from build123d import *

# Parameters (mm, degrees)
EXTRUDE_1_DEPTH      = 6
SKETCH_2_R           = 11.05
SKETCH_2_R_2         = 1.6
SKETCH_2_R_3         = 2.55
CUT_EXTRUDE_1_DEPTH  = 7
EXTRUDE_2_DEPTH      = 6
SKETCH_3_R           = 2.1
SKETCH_3_W           = 7
SKETCH_3_H           = 6
CUT_EXTRUDE_11_DEPTH = 7
EXTRUDE_21_DEPTH     = 6
SKETCH_31_R          = 2.1
SKETCH_31_W          = 7
SKETCH_31_H          = 6
CUT_EXTRUDE_12_DEPTH = 7
EXTRUDE_24_DEPTH     = 6
SKETCH_34_R          = 2.1
SKETCH_34_W          = 7
SKETCH_34_H          = 6
CUT_EXTRUDE_15_DEPTH = 7


with BuildPart() as part:
    # Эскиз1 → Бобышка-Вытянуть1 (new body)
    with BuildSketch(Plane.XY):
        with BuildLine():
            Line((0, -293.846153846), (66, -293.846153846))
            Line((66, -293.846153846), (66, -368.846153846))
            ThreePointArc((66, -368.846153846), (63.071067812, -375.917221658), (56, -378.846153846))
            Line((56, -378.846153846), (0, -378.846153846))
            Line((0, -378.846153846), (0, -293.846153846))
        make_face()
    extrude(amount=-EXTRUDE_1_DEPTH)

    # Эскиз2 → Вырез-Вытянуть1 (cut, through all)
    with BuildSketch(Plane.XY):
        with Locations((29, -353.846153846)):
            Circle(SKETCH_2_R)
        with Locations((44.5, -369.346153846)):
            Circle(SKETCH_2_R_2)
        with Locations((13.5, -369.346153846)):
            Circle(SKETCH_2_R_2)
        with Locations((13.5, -338.346153846)):
            Circle(SKETCH_2_R_2)
        with Locations((44.5, -338.346153846)):
            Circle(SKETCH_2_R_2)
        with Locations((29, -323.846153846)):
            Circle(SKETCH_2_R_3)
    extrude(amount=-CUT_EXTRUDE_1_DEPTH, mode=Mode.SUBTRACT)

    # Эскиз21 → Бобышка-Вытянуть2 (add)
    with BuildSketch(Plane(origin=(16, -335.846153846, 0), x_dir=(0, 1, 0), z_dir=(0, 0, -1))):
        with BuildLine():
            Line((13, 53), (-13, 53))
            ThreePointArc((-13, 53), (-14.118033989, 52.736067977), (-15, 52))
            Line((-15, 52), (-16.2, 50.4))
            ThreePointArc((-16.2, 50.4), (-16.552786405, 50.105572809), (-17, 50))
            Line((-17, 50), (17, 50))
            ThreePointArc((17, 50), (16.552786405, 50.105572809), (16.2, 50.4))
            Line((16.2, 50.4), (15, 52))
            ThreePointArc((15, 52), (14.118033989, 52.736067977), (13, 53))
        make_face()
    extrude(amount=EXTRUDE_2_DEPTH)

    # Эскиз3 → Вырез-Вытянуть11 (cut, through all)
    with BuildSketch(Plane(origin=(16, -335.846153846, -6), x_dir=(0, 1, 0), z_dir=(0, 0, -1))):
        with Locations((0, 47)):
            Circle(SKETCH_3_R)
        with Locations((9.531849908, 47)):
            Rectangle(SKETCH_3_W, SKETCH_3_H)
        with Locations((-9.531849908, 47)):
            Rectangle(SKETCH_3_W, SKETCH_3_H)
    extrude(amount=-CUT_EXTRUDE_11_DEPTH, mode=Mode.SUBTRACT)

    # Эскиз22 → Бобышка-Вытянуть21 (add)
    with BuildSketch(Plane(origin=(50, -310.846153846, 0), x_dir=(0, -1, 0), z_dir=(0, 0, -1))):
        with BuildLine():
            Line((13, 53), (-13, 53))
            ThreePointArc((-13, 53), (-14.118033989, 52.736067977), (-15, 52))
            Line((-15, 52), (-16.2, 50.4))
            ThreePointArc((-16.2, 50.4), (-16.552786405, 50.105572809), (-17, 50))
            Line((-17, 50), (17, 50))
            ThreePointArc((17, 50), (16.552786405, 50.105572809), (16.2, 50.4))
            Line((16.2, 50.4), (15, 52))
            ThreePointArc((15, 52), (14.118033989, 52.736067977), (13, 53))
        make_face()
    extrude(amount=EXTRUDE_21_DEPTH)

    # Эскиз31 → Вырез-Вытянуть12 (cut, through all)
    with BuildSketch(Plane(origin=(50, -310.846153846, -6), x_dir=(0, -1, 0), z_dir=(0, 0, -1))):
        with Locations((0, 47)):
            Circle(SKETCH_31_R)
        with Locations((9.531849908, 47)):
            Rectangle(SKETCH_31_W, SKETCH_31_H)
        with Locations((-9.531849908, 47)):
            Rectangle(SKETCH_31_W, SKETCH_31_H)
    extrude(amount=-CUT_EXTRUDE_12_DEPTH, mode=Mode.SUBTRACT)

    # Эскиз24 → Бобышка-Вытянуть24 (add)
    with BuildSketch(Plane(origin=(50, -361.846153846, 0), x_dir=(0, -1, 0), z_dir=(0, 0, -1))):
        with BuildLine():
            Line((13, 53), (-13, 53))
            ThreePointArc((-13, 53), (-14.118033989, 52.736067977), (-15, 52))
            Line((-15, 52), (-16.2, 50.4))
            ThreePointArc((-16.2, 50.4), (-16.552786405, 50.105572809), (-17, 50))
            Line((-17, 50), (17, 50))
            ThreePointArc((17, 50), (16.552786405, 50.105572809), (16.2, 50.4))
            Line((16.2, 50.4), (15, 52))
            ThreePointArc((15, 52), (14.118033989, 52.736067977), (13, 53))
        make_face()
    extrude(amount=EXTRUDE_24_DEPTH)

    # Эскиз34 → Вырез-Вытянуть15 (cut, through all)
    with BuildSketch(Plane(origin=(50, -361.846153846, -6), x_dir=(0, -1, 0), z_dir=(0, 0, -1))):
        with Locations((0, 47)):
            Circle(SKETCH_34_R)
        with Locations((9.531849908, 47)):
            Rectangle(SKETCH_34_W, SKETCH_34_H)
        with Locations((-9.531849908, 47)):
            Rectangle(SKETCH_34_W, SKETCH_34_H)
    extrude(amount=-CUT_EXTRUDE_15_DEPTH, mode=Mode.SUBTRACT)


solid = part.part
Work out the finished part from the listing and answer in its coordinate system (mm). A direction names the side the tool comes from. Coordinates: 2 decimals unless noted, no trailing zeros. Write each loop counter-clockwise with the first axis right and the second up, starting at its lowest first coordinate (ties: lowest second). Pieces come first, ordered by that corner, then holes. Notation, with made-up numbers: M 21.5,20.5 L 33.5,20.5 A23 cw 33.5,45.5 Z; hole C 27,-40 d7. An arc over 180 degrees is marked long. Use one line per item in the form item = value. Start each with the question number.
1. The part is cut by section A-A (x = 3). Give the vertices of the cut face in (y, z), plus the area to 3 significant figures.
2. The mould has two halves that part along Y. Classify faces 3 (the face through (3, -355.814, -3)), 4 (the face through (-3, -362, -3)), 5 (the face through (63.15, -375.84, -2.96)): released by +Y, released by -Y, zero draft, split by the parting line, or undercut.
3. Each of these flat-tipped pins is pushed along its axis until it touches: P1, Ø1.8, axis at y = -327.5, z = -3, coming from the -X side; P2, Ø20, axis at x = 29, y = -353.85, coming from the -Z side; P3, Ø1, axis at y = -353.5, z = -4.5, coming from the +X side; P4, Ø3, axis at x = 63.5, z = -2, coming from the -Y side. Where does it stop, or does it pass through?
4. The part is cut by section C-C (x = 63). Give the vertices of the cut face in (y, z), plus the area to 3 significant figures.
5. A tool of negligible diameter and unlimited length cuts with its end or side. For faces 1 (the face through (68.729, -321.714, -2.958)), 2 (the face through (66, -326, -3)), from which of +Z, -Z, +X, -X, +Y, -Y can it reach the whole face along a straight path? Write none if from no direction.
6. The part is cut by section D-D (z = -2.9). Give the number of separate pieces and of enclosed holes in the cut face, plus the area to 3 significant figures.
7. The part is cut by section B-B (x = 29). Give the vertices of the cut face in (y, z).
8. Straight lines are drawn through the part: probe 1 along X at (y, z) = (-354.5, -3.5); probe 2 along X at (y, z) = (-369.5, -1.65); probe 3 along Y at (x, z) = (45, -4.4). For each, find the intervals that lie inside material, in ascending order. Write a range as from..to.
Evaluation:
q1.outline = M -378.85,-6 L -374.88,-6 L -374.88,0 L -378.85,0 Z; M -367.88,-6 L -363.95,-6 L -363.95,0 L -367.88,0 Z; M -359.75,-6 L -355.81,-6 L -355.81,0 L -359.75,0 Z; M -348.81,-6 L -323.88,-6 L -323.88,0 L -348.81,0 Z; M -316.88,-6 L -312.95,-6 L -312.95,0 L -316.88,0 Z; M -308.75,-6 L -304.81,-6 L -304.81,0 L -308.75,0 Z; M -297.81,-6 L -293.85,-6 L -293.85,0 L -297.81,0 Z
q1.area = 292 mm^2
q2.face_3 = undercut
q2.face_4 = zero draft
q2.face_5 = released by -Y
q3.P1 = -0.99
q3.P2 = through
q3.P3 = 66
q3.P4 = -376.85
q4.outline = M -375.99,-6 L -348.88,-6 L -348.88,0 L -375.99,0 Z; M -341.88,-6 L -337.95,-6 L -337.95,0 L -341.88,0 Z; M -333.75,-6 L -329.81,-6 L -329.81,0 L -333.75,0 Z; M -322.81,-6 L -293.85,-6 L -293.85,0 L -322.81,0 Z
q4.area = 384 mm^2
q5.face_1 = +Z, -Z, +X, +Y
q5.face_2 = +Z, -Z
q6.separate_pieces = 1
q6.enclosed_holes = 15
q6.area = 5,130 mm^2
q7.outline = M -378.85,-6 L -364.9,-6 L -364.9,0 L -378.85,0 Z; M -342.8,-6 L -326.4,-6 L -326.4,0 L -342.8,0 Z; M -321.3,-6 L -293.85,-6 L -293.85,0 L -321.3,0 Z
q8.probe_1 = -3..0, 6..17.97, 40.03..66
q8.probe_2 = -3..0, 6..11.91, 15.09..42.91, 46.09..65.98
q8.probe_3 = -378.85..-370.87, -367.83..-339.87, -336.83..-293.85
